Solid Edge part; units mm, degrees
sketch "Sketch1" plane through (0, 0, 8) normal (0, 0, 1) x (1, 0, 0)
  circle A0 centre (0, 0) radius 21
  circle A1 centre (0, 0) radius 12
  circle A2 centre (11.3137, 11.3137) radius 1.7
  circle A3 centre (-11.3137, 11.3137) radius 1.7
  circle A4 centre (-11.3137, -11.3137) radius 1.7
  circle A5 centre (11.3137, -11.3137) radius 1.7
extrude "ExtrudedProtrusion_1" add sketch "Sketch1" along normal blind 4
sketch "Sketch2" plane through (0, 0, 8) normal (0, 0, 1) x (1, 0, 0)
  line L0 (12, -12) -> (73, -12)
  line L1 (73, -12) -> (73, 12)
  line L2 (73, 12) -> (12, 12)
  line L3 (12, 12) -> (12, -12)
extrude "ExtrudedProtrusion_2" add sketch "Sketch2" along normal blind 4
sketch "Sketch3" plane through (0, 0, 8) normal (0, 0, 1) x (1, 0, 0)
  line L0 (57, -49) -> (113, -49)
  line L1 (113, -49) -> (113, 24)
  line L2 (113, 24) -> (57, 24)
  line L3 (57, 24) -> (57, -49)
  circle A0 centre (62, -43) radius 1.7
  circle A1 centre (108, -43) radius 1.7
  circle A2 centre (62, 18) radius 1.7
  circle A3 centre (108, 18) radius 1.7
extrude "ExtrudedProtrusion_3" add sketch "Sketch3" along normal blind 4
Design review of the part built by this model. Coordinates are the model's own, in mm. A direction names the side the tool comes from. Round coordinates to 2 decimals unless told otherwise and drop trailing zeros. Write each loop counter-clockwise with the first axis right and the second up, starting at its lowest first coordinate (ties: lowest second). Pieces come first, ordered by that corner, then holes. Notation, with made-up numbers: (48, 52) -> (56, 52) arc R14 ccw to (56, 62) -> close; hole circle Ø8 at (-9, 75.5). An arc over 180 degrees is marked (long way). Answer in a Markdown table with one row per item.
Q1. Take a section at C-C, the plane x = 62. State the section outline as (y, z) points, then the cut area to 3 significant figures.
The answers:
| item | result |
|---|---|
| outline | (-49, 8) -> (-44.7, 8) -> (-44.7, 12) -> (-49, 12) -> close; (-41.3, 8) -> (16.3, 8) -> (16.3, 12) -> (-41.3, 12) -> close; (19.7, 8) -> (24, 8) -> (24, 12) -> (19.7, 12) -> close |
| area | 265 mm² |
Q2. Draft analysis for pull direction X (two halves, no side actions). For faces 4 (the face through (-11.99, -0.53, 9.97)), 5 (the face through (-9.743, -10.663, 9.972)), 6 (the face through (60, -12, 12)), 7 (the face through (113, -13, 10)), state which applies: +X half, -X half, draft (parallel to the pull), parting line (faces both ways), or undercut.
The answers:
| item | result |
|---|---|
| face 4 | undercut |
| face 5 | undercut |
| face 6 | draft |
| face 7 | +X half |
Q3. Take a section at B-B, the plane x = 0. State the section outline as (y, z) points.
The answers:
| item | result |
|---|---|
| outline | (-21, 8) -> (-12, 8) -> (-12, 12) -> (-21, 12) -> close; (12, 8) -> (21, 8) -> (21, 12) -> (12, 12) -> close |
Q4. Take a section at D-D, the plane y = -43. State the section outline as (x, z) points, then the cut area to 3 significant figures.
The answers:
| item | result |
|---|---|
| outline | (57, 8) -> (60.3, 8) -> (60.3, 12) -> (57, 12) -> close; (63.7, 8) -> (106.3, 8) -> (106.3, 12) -> (63.7, 12) -> close; (109.7, 8) -> (113, 8) -> (113, 12) -> (109.7, 12) -> close |
| area | 197 mm² |
Q5. For faces 1 (the face through (37, 12, 10)), 2 (the face through (57, -30, 10)), 3 (the face through (60.65, -41.97, 9.97)), list the 3-axis set-ups (+Z, -Z, +X, -X, +Y, -Y) from which the entire face can be reached by the end or side of a thin tool; tool diameter is ignored.
The answers:
| item | result |
|---|---|
| face 1 | +Z, -Z, +Y |
| face 2 | +Z, -Z, -Y |
| face 3 | +Z, -Z |
Q6. To check wall thickness, follow L1, parallel to X at y = 18.5, z = 8.3; L2, parallel to Y at x = 106.5, z = 9.55; L3, parallel to X at y = -29.5, z = 11.2. State the ranges of each line that lie inside material, in increasing order. Write a range as [from, to].
The answers:
| item | result |
|---|---|
| L1 | [-9.94, 9.94], [57, 60.38], [63.62, 106.38], [109.62, 113] |
| L2 | [-49, -43.8], [-42.2, 17.2], [18.8, 24] |
| L3 | [57, 113] |
Q7. Take a section at A-A, the plane y = 0. State the section outline as (x, z) points, then the cut area to 3 significant figures.
The answers:
| item | result |
|---|---|
| outline | (-21, 8) -> (-12, 8) -> (-12, 12) -> (-21, 12) -> close; (12, 8) -> (113, 8) -> (113, 12) -> (12, 12) -> close |
| area | 440 mm² |
Q8. Clearance check with flat-ended pins moving along their axes: pin 1 Ø4 at (x, y) = (62, -43) entering from +Z; pin 2 Ø0.7 at (y, z) = (10.5, 11) entering from -X; pin 3 Ø1.2 at (y, z) = (-24.5, 9.5) entering from -X. State where each tip first meets the part, or that it passes through.
The answers:
| item | result |
|---|---|
| pin 1 | z = 12 |
| pin 2 | x = -18.38 |
| pin 3 | x = 57 |
